```python
from build123d import *
from build123d.topology import SkipClean

# Parameters (mm, degrees)
SKETCH_1_R          = 1.50000254
EXTRUDE_1_DEPTH     = 1.5
EXTRUDE_START       = 5.4999492
SKETCH_2_R          = 5.479431536
EXTRUDE_2_DEPTH     = 5.4999492
SKETCH_3_R          = 2
SKETCH_3_R_2        = 1
CUT_EXTRUDE_1_DEPTH = 1.5
SKETCH_4_W          = 28
SKETCH_4_H          = 20.5
CUT_EXTRUDE_2_DEPTH = 1.5
SKETCH_5_R          = 1.50000254
EXTRUDE_3_DEPTH     = 5.4999492
SKETCH_7_W          = 30.2
SKETCH_7_H          = 22.7
CUT_EXTRUDE_3_DEPTH = 1.5
SKETCH_8_R          = 1.517681864
EXTRUDE_5_DEPTH     = 0.524949197
SKETCH_10_W         = 30.2
SKETCH_10_H         = 27.8
CUT_EXTRUDE_5_DEPTH = 1.1
SKETCH_6_R          = 1
SKETCH_6_R_2        = 2
SKETCH_6_W          = 28
SKETCH_6_H          = 20.5
EXTRUDE_4_DEPTH     = 0.2
CUT_EXTRUDE_4_DEPTH = 14.2
SKETCH_13_R         = 1.517681864
CUT_EXTRUDE_8_DEPTH = 0.7
SKETCH_11_R         = 1.50000254
CUT_EXTRUDE_6_DEPTH = 1.7
SKETCH_12_R         = 2.6
CUT_EXTRUDE_7_DEPTH = 2.5
SKETCH_14_W         = 1.6
SKETCH_14_H         = 8
CUT_EXTRUDE_9_DEPTH = 1.5


with BuildPart() as part:
    # 草图1 → 凸台-拉伸1 (new body)
    with BuildSketch(Plane.XY.offset(7.1)):
        with BuildLine():
            Line((-1.187299975, -2.77233639), (-1.187299975, -32.77239481))
            ThreePointArc((-1.187299975, -32.77239481), (0.624921207, -37.147483764), (5.00001016, -38.959704945))
            Line((5.00001016, -38.959704945), (55.00010922, -38.959704945))
            ThreePointArc((55.00010922, -38.959704945), (59.375198174, -37.147483764), (61.187419355, -32.77239481))
            Line((61.187419355, -32.77239481), (61.187419355, -2.77233639))
            ThreePointArc((61.187419355, -2.77233639), (59.375198174, 1.602752563), (55.00010922, 3.414973745))
            Line((55.00010922, 3.414973745), (5.00001016, 3.414973745))
            ThreePointArc((5.00001016, 3.414973745), (0.624921207, 1.602752563), (-1.187299975, -2.77233639))
        make_face()
        with Locations((56.50012446, -1.27234401)):
            Circle(SKETCH_1_R, mode=Mode.SUBTRACT)
        with Locations((56.50011176, -34.27239989)):
            Circle(SKETCH_1_R, mode=Mode.SUBTRACT)
        with Locations((3.50000762, -34.27239989)):
            Circle(SKETCH_1_R, mode=Mode.SUBTRACT)
        with Locations((3.50002286, -1.27236433)):
            Circle(SKETCH_1_R, mode=Mode.SUBTRACT)
    extrude(amount=EXTRUDE_1_DEPTH)

    # 草图2 → 凸台-拉伸2 (add)
    with BuildSketch(Plane(origin=(0, 0, 7.1), x_dir=(-1, 0, 0), z_dir=(0, 0, -1)).offset(EXTRUDE_START)):
        with BuildLine():
            ThreePointArc((-55.085589107, -33.773267358), (-45.891997384, -24.658833945), (-55.864584942, -32.913682376))
            ThreePointArc((-55.864584942, -32.913682376), (-55.388627485, -33.265121217), (-55.085589107, -33.773267358))
        make_face()
        with Locations((-50.693180097, -29.009888712)):
            Circle(SKETCH_2_R, mode=Mode.SUBTRACT)
    extrude(amount=-EXTRUDE_2_DEPTH)

    # 草图3 → 切除-拉伸1 (cut)
    with BuildSketch(Plane(origin=(0, 0, 7.1), x_dir=(-1, 0, 0), z_dir=(0, 0, -1))):
        with Locations((-50.693180097, -29.009888712)):
            Circle(SKETCH_3_R)
        with Locations((-54.493180097, -29.009888712)):
            Circle(SKETCH_3_R_2)
        with Locations((-50.693180097, -25.209888712)):
            Circle(SKETCH_3_R_2)
        with Locations((-46.893180097, -29.009888712)):
            Circle(SKETCH_3_R_2)
        with Locations((-50.693180097, -32.809888712)):
            Circle(SKETCH_3_R_2)
    extrude(amount=-CUT_EXTRUDE_1_DEPTH, mode=Mode.SUBTRACT)

    # 草图4 → 切除-拉伸2 (cut)
    with BuildSketch(Plane.XY.offset(8.6)):
        with Locations((20.00004064, -17.77236687)):
            Rectangle(SKETCH_4_W, SKETCH_4_H)
    extrude(amount=-CUT_EXTRUDE_2_DEPTH, mode=Mode.SUBTRACT)

    # 草图5 → 凸台-拉伸3 (add)
    # profile 1 of 4: a face of its own
    with SkipClean():  # the faces are left unmerged after this step: merging them gives an invalid solid
        with BuildSketch(Plane(origin=(0, 0, 7.1), x_dir=(-1, 0, 0), z_dir=(0, 0, -1)).offset(EXTRUDE_START)):
            with BuildLine():
                Line((-60.187419355, -2.77233639), (-60.187419355, -4.27234401))
                Line((-60.187419355, -4.27234401), (-56.50012446, -4.27234401))
                ThreePointArc((-56.50012446, -4.27234401), (-54.378804117, -3.393664354), (-53.50012446, -1.27234401))
                Line((-53.50012446, -1.27234401), (-53.50012446, 2.414973745))
                Line((-53.50012446, 2.414973745), (-55.00010922, 2.414973745))
                ThreePointArc((-55.00010922, 2.414973745), (-58.668091393, 0.895645782), (-60.187419355, -2.77233639))
            make_face()
            with Locations((-56.50012446, -1.27234401)):
                Circle(SKETCH_5_R, mode=Mode.SUBTRACT)
        # profile 2 of 4: a face of its own
        with BuildSketch(Plane(origin=(0, 0, 7.1), x_dir=(-1, 0, 0), z_dir=(0, 0, -1)).offset(EXTRUDE_START)):
            with BuildLine():
                ThreePointArc((-54.137667628, -34.27239989), (-54.829611494, -32.601899624), (-56.50011176, -31.909955757))
                Line((-56.50011176, -31.909955757), (-60.187419355, -31.909955757))
                Line((-60.187419355, -31.909955757), (-60.187419355, -32.77239481))
                ThreePointArc((-60.187419355, -32.77239481), (-58.668091393, -36.440376982), (-55.00010922, -37.959704945))
                Line((-55.00010922, -37.959704945), (-54.137667628, -37.959704945))
                Line((-54.137667628, -37.959704945), (-54.137667628, -34.27239989))
            make_face()
            with Locations((-56.50011176, -34.27239989)):
                Circle(SKETCH_5_R, mode=Mode.SUBTRACT)
        # profile 3 of 4: a face of its own
        with BuildSketch(Plane(origin=(0, 0, 7.1), x_dir=(-1, 0, 0), z_dir=(0, 0, -1)).offset(EXTRUDE_START)):
            with BuildLine():
                Line((-6.50002286, -34.27236687), (-6.50002286, -37.959704945))
                Line((-6.50002286, -37.959704945), (-5.00001016, -37.959704945))
                ThreePointArc((-5.00001016, -37.959704945), (-1.332027988, -36.440376982), (0.187299975, -32.77239481))
                Line((0.187299975, -32.77239481), (0.187299975, -31.27236687))
                Line((0.187299975, -31.27236687), (-3.50002286, -31.27236687))
                ThreePointArc((-3.50002286, -31.27236687), (-5.621343204, -32.151046526), (-6.50002286, -34.27236687))
            make_face()
            with Locations((-3.50000762, -34.27239989)):
                Circle(SKETCH_5_R, mode=Mode.SUBTRACT)
        # profile 4 of 4: a face of its own
        with BuildSketch(Plane(origin=(0, 0, 7.1), x_dir=(-1, 0, 0), z_dir=(0, 0, -1)).offset(EXTRUDE_START)):
            with BuildLine():
                Line((-5.00001016, 2.414973745), (-6.50002286, 2.414973745))
                Line((-6.50002286, 2.414973745), (-6.50002286, -1.27236433))
                ThreePointArc((-6.50002286, -1.27236433), (-5.621343204, -3.393684674), (-3.50002286, -4.27236433))
                Line((-3.50002286, -4.27236433), (0.187299975, -4.27236433))
                Line((0.187299975, -4.27236433), (0.187299975, -2.77233639))
                ThreePointArc((0.187299975, -2.77233639), (-1.332027988, 0.895645782), (-5.00001016, 2.414973745))
            make_face()
            with Locations((-3.50002286, -1.27236433)):
                Circle(SKETCH_5_R, mode=Mode.SUBTRACT)
        extrude(amount=-EXTRUDE_3_DEPTH)

    # 草图7 → 切除-拉伸3 (cut)
    with SkipClean():  # the faces are left unmerged after this step: merging them gives an invalid solid
        with BuildSketch(Plane.XY.offset(8.6)):
            with Locations((20.00004064, -17.77236687)):
                Rectangle(SKETCH_7_W, SKETCH_7_H)
        extrude(amount=-CUT_EXTRUDE_3_DEPTH, mode=Mode.SUBTRACT)

    # 草图8 → 凸台-拉伸5 (add)
    with SkipClean():  # the faces are left unmerged after this step: merging them gives an invalid solid
        with BuildSketch(Plane(origin=(0, 0, 7.1), x_dir=(-1, 0, 0), z_dir=(0, 0, -1))):
            with Locations(Location((-43.053086106, -19.36236941, 0), (0, 0, 180))):
                Circle(SKETCH_8_R)
        extrude(amount=EXTRUDE_5_DEPTH)

    # 草图10 → 切除-拉伸5 (cut)
    with SkipClean():  # the faces are left unmerged after this step: merging them gives an invalid solid
        with BuildSketch(Plane(origin=(0, 0, 7.1), x_dir=(-1, 0, 0), z_dir=(0, 0, -1))):
            with Locations((-20.00004064, -17.77236687)):
                Rectangle(SKETCH_10_W, SKETCH_10_H)
        extrude(amount=-CUT_EXTRUDE_5_DEPTH, mode=Mode.SUBTRACT)

    # 草图6 → 凸台-拉伸4 (add)
    with BuildSketch(Plane.XY.offset(8.6)):
        with BuildLine():
            Line((-1.187299975, -2.77233639), (-1.187299975, -32.77239481))
            ThreePointArc((-1.187299975, -32.77239481), (0.624921207, -37.147483764), (5.00001016, -38.959704945))
            Line((5.00001016, -38.959704945), (55.00010922, -38.959704945))
            ThreePointArc((55.00010922, -38.959704945), (59.375198174, -37.147483764), (61.187419355, -32.77239481))
            Line((61.187419355, -32.77239481), (61.187419355, -2.77233639))
            ThreePointArc((61.187419355, -2.77233639), (59.375198174, 1.602752563), (55.00010922, 3.414973745))
            Line((55.00010922, 3.414973745), (5.00001016, 3.414973745))
            ThreePointArc((5.00001016, 3.414973745), (0.624921207, 1.602752563), (-1.187299975, -2.77233639))
        make_face()
        with Locations(Location((46.893180097, -29.009888712, 0), (0, 0, 180))):
            Circle(SKETCH_6_R, mode=Mode.SUBTRACT)
        with Locations(Location((50.693180097, -32.809888712, 0), (0, 0, 180))):
            Circle(SKETCH_6_R, mode=Mode.SUBTRACT)
        with Locations(Location((54.493180097, -29.009888712, 0), (0, 0, 180))):
            Circle(SKETCH_6_R, mode=Mode.SUBTRACT)
        with Locations(Location((50.693180097, -29.009888712, 0), (0, 0, 180))):
            Circle(SKETCH_6_R_2, mode=Mode.SUBTRACT)
        with Locations(Location((50.693180097, -25.209888712, 0), (0, 0, 180))):
            Circle(SKETCH_6_R, mode=Mode.SUBTRACT)
        with Locations((20.00004064, -17.77236687)):
            Rectangle(SKETCH_6_W, SKETCH_6_H, mode=Mode.SUBTRACT)
    extrude(amount=EXTRUDE_4_DEPTH)

    # 草图9 → 切除-拉伸4 (cut)
    with BuildSketch(Plane(origin=(0, 0, 7.1), x_dir=(-1, 0, 0), z_dir=(0, 0, -1))):
        with BuildLine():
            Line((-43.053086106, -16.36236941), (-38.053086106, -16.36236941))
            Line((-38.053086106, -16.36236941), (-38.053086106, -15.86236941))
            Line((-38.053086106, -15.86236941), (-43.053086106, -15.86236941))
            ThreePointArc((-43.053086106, -15.86236941), (-46.553086106, -19.36236941), (-43.053086106, -22.86236941))
            Line((-43.053086106, -22.86236941), (-38.053086106, -22.86236941))
            Line((-38.053086106, -22.86236941), (-38.053086106, -22.36236941))
            Line((-38.053086106, -22.36236941), (-43.053086106, -22.36236941))
            ThreePointArc((-43.053086106, -22.36236941), (-46.053086106, -19.36236941), (-43.053086106, -16.36236941))
        make_face()
    extrude(amount=-CUT_EXTRUDE_4_DEPTH, mode=Mode.SUBTRACT)

    # 草图13 → 切除-拉伸8 (cut)
    with BuildSketch(Plane(origin=(0, 0, 7.1), x_dir=(-1, 0, 0), z_dir=(0, 0, -1))):
        with BuildLine():
            Line((-43.053086106, -16.36236941), (-38.053086106, -16.36236941))
            Line((-38.053086106, -16.36236941), (-37.253086106, -16.36236941))
            Line((-37.253086106, -16.36236941), (-37.253086106, -22.36236941))
            Line((-37.253086106, -22.36236941), (-38.053086106, -22.36236941))
            Line((-38.053086106, -22.36236941), (-43.053086106, -22.36236941))
            ThreePointArc((-43.053086106, -22.36236941), (-46.053086106, -19.36236941), (-43.053086106, -16.36236941))
        make_face()
        with Locations(Location((-43.053086106, -19.36236941, 0), (0, 0, 180))):
            Circle(SKETCH_13_R, mode=Mode.SUBTRACT)
    extrude(amount=-CUT_EXTRUDE_8_DEPTH, mode=Mode.SUBTRACT)

    # 草图11 → 切除-拉伸6 (cut)
    with BuildSketch(Plane(origin=(0, 0, 7.1), x_dir=(-1, 0, 0), z_dir=(0, 0, -1))):
        with Locations((-56.50012446, -1.27234401)):
            Circle(SKETCH_11_R)
        with Locations((-3.50002286, -1.27236433)):
            Circle(SKETCH_11_R)
        with Locations((-56.50011176, -34.27239989)):
            Circle(SKETCH_11_R)
        with Locations((-3.50000762, -34.27239989)):
            Circle(SKETCH_11_R)
    extrude(amount=-CUT_EXTRUDE_6_DEPTH, mode=Mode.SUBTRACT)

    # 草图12 → 切除-拉伸7 (cut)
    with BuildSketch(Plane.XY.offset(8.8)):
        with Locations((3.50002286, -1.27236433)):
            Circle(SKETCH_12_R)
        with Locations(Location((56.50009652, -1.27236433, 0), (0, 0, 180))):
            Circle(SKETCH_12_R)
        with Locations((56.50009652, -34.27236687)):
            Circle(SKETCH_12_R)
        with Locations(Location((3.50002286, -34.27236687, 0), (0, 0, 180))):
            Circle(SKETCH_12_R)
    extrude(amount=-CUT_EXTRUDE_7_DEPTH, mode=Mode.SUBTRACT)

    # 草图14 → 切除-拉伸9 (cut)
    with BuildSketch(Plane(origin=(0, 0, 7.1), x_dir=(-1, 0, 0), z_dir=(0, 0, -1))):
        with Locations((-4.90004064, -17.7723656)):
            Rectangle(SKETCH_14_W, SKETCH_14_H)
    extrude(amount=-CUT_EXTRUDE_9_DEPTH, mode=Mode.SUBTRACT)


solid = part.part
```
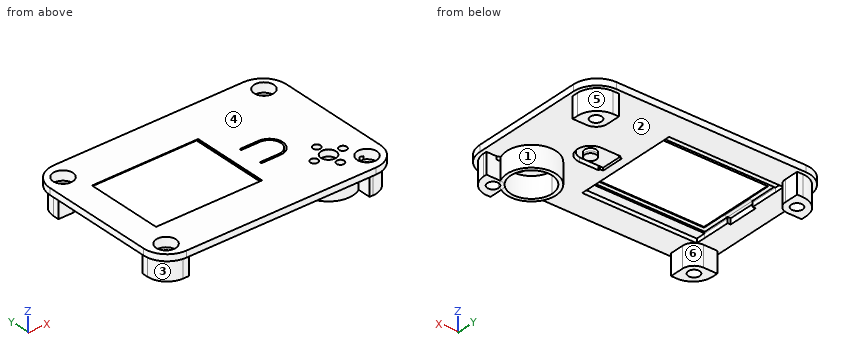
Work out the finished part from the listing and answer in its coordinate system (mm). Face numbers are marked on the shaded views. A direction names the side the tool comes from. Give positions to 0.01 mm unless a question says otherwise; leave off trailing zeros. Loops run counter-clockwise (first coordinate to the right, second up) from the corner with the lowest first, then second, coordinate; pieces in that order, holes last. Notation, with made-up numbers: M 69.5,-1 L 101.5,-1 A14 cw 101.5,26 Z; hole C 82.25,27.5 d5. An arc over 180 degrees is marked long. One line per item, written item: value. Start each with the question number.
1. Find section C-C (y = -20). Give the vertices of the cut face in (x, z), and give its area (3 significant figures).
2. Find section B-B (x = 11). Give the vertices of the cut face in (y, z), and give its area (3 significant figures).
3. Find the intervals of material crossed by probe 1 along Y at (x, z) = (40, 8); probe 2 along Y at (x, z) = (7.5, 8.25); probe 3 along X at (y, z) = (-8, 8), in increasing order.
4. Which of the six approach directions +Z, -Z, +X, -X, +Y, -Y give full straight-line access (tool end or side, diameter ignored) to the marked faces 5 and 6?
5. Find section D-D (y = -13). Give the vertices of the cut face in (x, z).
6. Each of these flat-tipped pins is pushed along its axis until it touches: P1, Ø0.5, axis at x = 5.5, z = 5, coming from the +Y side (3 decimals); P2, Ø1.5, axis at x = 17.5, z = 6.5, coming from the +Y side (3 decimals); P3, Ø5, axis at x = 23.5, y = -4, coming from the -Z side; P4, Ø18, axis at x = 25, y = -22.5, coming from the -Z side. Where does it stop, or does it pass through?
7. Determine the mould class of the marked faces 1, 2, 3 and 4 for opening direction X: released by +X, released by -X, zero draft, split by the parting line, or undercut.
8. Find section A-A (z = 2.5). State how many separate pieces and enclosed holes the cut face has, and give its area (3 significant figures).
Reported:
1. outline: M -1.19,7.1 L 4.1,7.1 L 4.1,8.6 L 6,8.6 L 6,8.8 L -1.19,8.8 Z; M 34,8.6 L 35.1,8.6 L 35.1,7.1 L 37.25,7.1 L 37.25,7.8 L 41.68,7.8 L 41.68,6.58 L 44.43,6.58 L 44.43,7.8 L 45.98,7.8 L 45.98,8.8 L 34,8.8 Z; M 46.49,7.1 L 61.19,7.1 L 61.19,8.8 L 46.49,8.8 Z
1. area: 50.3 mm²
2. outline: M -38.96,7.1 L -31.67,7.1 L -31.67,8.2 L -29.12,8.2 L -29.12,8.6 L -28.02,8.6 L -28.02,8.8 L -38.96,8.8 Z; M -7.52,8.6 L -6.42,8.6 L -6.42,8.2 L -3.87,8.2 L -3.87,7.1 L 3.41,7.1 L 3.41,8.8 L -7.52,8.8 Z
2. area: 28.3 mm²
3. probe 1: y = -38.96 to -22.86, -22.36 to -16.36, -15.86 to 3.41
3. probe 2: y = -38.96 to -29.12, -6.42 to 3.41
3. probe 3: x = -1.19 to 4.9, 35.1 to 61.19
4. face 5: -Z, +X, +Y
4. face 6: -Z
5. outline: M -1.19,7.1 L 4.9,7.1 L 4.9,8.6 L 6,8.6 L 6,8.8 L -1.19,8.8 Z; M 34,8.6 L 35.1,8.6 L 35.1,7.1 L 61.19,7.1 L 61.19,8.8 L 34,8.8 Z
6. P1: stops at y = 2.415
6. P2: stops at y = 3.415
6. P3: stops at z = 7.1
6. P4: stops at z = 8.2
7. face 1: undercut
7. face 2: undercut
7. face 3: released by -X
7. face 4: zero draft
8. separate pieces: 4
8. enclosed holes: 5
8. area: 148 mm²
